```python
from build123d import *

# Parameters (mm, degrees)
SKICA1_R                 = 20
P_IDAT_VYSUNUT_M1_DEPTH  = 60
SKICA2_R                 = 2.075
ODEBRAT_VYSUNUT_M1_DEPTH = 60
SKICA3_R                 = 4
ODEBRAT_VYSUNUT_M2_DEPTH = 35
ZKOSEN_1_SIZE            = 0.5


with BuildPart() as part:
    # Skica1 → Přidat vysunutím1 (new body)
    with BuildSketch(Plane.XY):
        Circle(SKICA1_R)
    extrude(amount=P_IDAT_VYSUNUT_M1_DEPTH)

    # Skica2 → Odebrat vysunutím1 (cut)
    with BuildSketch(Plane.XY.offset(60)):
        Circle(SKICA2_R)
    extrude(amount=-ODEBRAT_VYSUNUT_M1_DEPTH, mode=Mode.SUBTRACT)

    # Skica3 → Odebrat vysunutím2 (cut)
    with BuildSketch(Plane.XY.offset(60)):
        Circle(SKICA3_R)
    extrude(amount=-ODEBRAT_VYSUNUT_M2_DEPTH, mode=Mode.SUBTRACT)

    # Zkosení1
    zkosen_1_edges = [part.edges().sort_by_distance(p)[0] for p in [
        (-2.075, 0, 25),
    ]]
    chamfer(zkosen_1_edges, length=ZKOSEN_1_SIZE)


solid = part.part
```
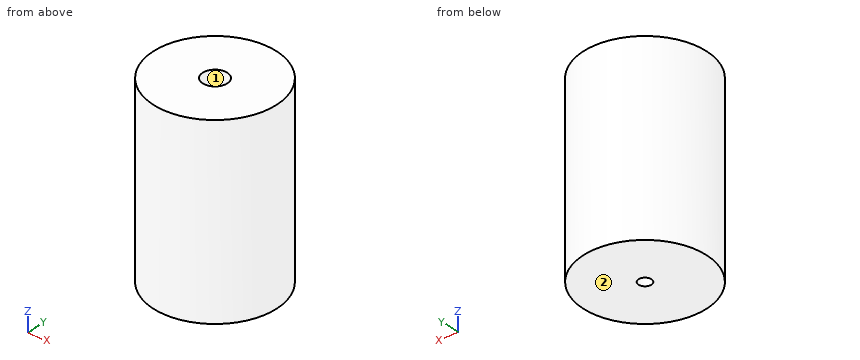
For this review, take the finished solid that the model builds, in its own axes (mm). Face numbers are marked on the shaded views. A direction names the side the tool comes from. Give positions to 0.01 mm unless a question says otherwise; leave off trailing zeros. Loops run counter-clockwise (first coordinate to the right, second up) from the corner with the lowest first, then second, coordinate; pieces in that order, holes last. Notation, with made-up numbers: M 61,-2.75 L 97,-2.75 A17 cw 97,2.25 Z; hole C 37,-10 d10. An arc over 180 degrees is marked long. One line per item, written item: value. Start each with the question number.
Q1. Add section C-C (z = 34). Give the boundary of the cut face in (x, y), and give its area (3 significant figures).
Q2. Add section D-D (y = 16). Give the boundary of the cut face in (x, z).
Q3. Clearance check with flat-ended pins moving along their axes: pin 1 Ø7 at (x, y) = (0, 0) entering from +Z; pin 2 Ø2 at (y, z) = (2, 36.5) entering from +X (3 decimals); pin 3 Ø1.5 at (y, z) = (4.5, 33) entering from -X; pin 4 Ø2.5 at (x, y) = (0, 0) entering from +Z. State where each tip first meets the part, or that it passes through.
Q4. Add section A-A (y = 0). Give the boundary of the cut face in (x, z) (3 decimals).
Q5. For L1, parallel to Y at x = 0, z = 32; L2, parallel to Y at x = 0, z = 10.75 (3 decimals); L3, parallel to X at y = -2, z = 43, list the stretches that pass through material, from the lowest coordinate up.
Q6. Machinability: for the marked faces 1 and 2, which of the approach directions +Z, -Z, +X, -X, +Y, -Y give a long, thin tool a straight path to every point of the face, cutting with its end or side? Answer none if there is none.
Reply:
1. outline: C 0,0 d40; hole C 0,0 d8
1. area: 1,210 mm²
2. outline: M -12,0 L 12,0 L 12,60 L -12,60 Z
3. pin 1: z = 25
3. pin 2: x = 19.975
3. pin 3: x = -19.65
3. pin 4: through
4. outline: M -20,0 L -2.075,0 L -2.075,24.5 L -2.575,25 L -4,25 L -4,60 L -20,60 Z; M 2.075,0 L 20,0 L 20,60 L 4,60 L 4,25 L 2.575,25 L 2.075,24.5 Z
5. L1: -20 to -4, 4 to 20
5. L2: -20 to -2.075, 2.075 to 20
5. L3: -19.9 to -3.46, 3.46 to 19.9
6. face 1: +Z
6. face 2: -Z, +X, -X, +Y, -Y
